Can you work these out from the model? Positions are in its coordinate system, mm. A direction names the side the tool comes from. Round coordinates to 2 decimals unless told otherwise and drop trailing zeros. Order: outer loops, then holes, each group sorted by start corner. A loop starts at its lowest first (then second) coordinate and runs counter-clockwise, first axis right, second up.
Q1. If we section it at B-B (x = -55.5): Please give me the cut outline in (y, z), plus the area to 3 significant figures.
Q2. If we section it at D-D (y = -8.5): Please give me the cut outline in (x, z), plus the area to 3 significant figures.
Q3. If we section it at A-A (z = -10): Please give me the cut outline in (x, y), plus the area to 3 significant figures.
Q4. We'd pull the mould along Y, two halves only. Please class faces 1 (the face through (-21, 82.55, -27)), 2 (the face through (-22, 0, -17)), 3 (the face through (-6, -9, 0)), 4 (the face through (-22, -19.05, -27)): pulls with the +Y half, pulls with the -Y half, needs draft (parallel to the pull), parting line crosses it, or undercut.
Q5. Will these pins go through, and if not, where does the flat tip stop? P1, Ø13.5, axis at x = -21, y = 28.5, coming from the +Z side; P2, Ø6, axis at y = -1, z = -17, coming from the -X side; P3, Ø15, axis at y = 38, z = -31.5, coming from the -X side.
Q6. If I drill on line 1 (Y direction, x = -57.5, z = -32); line 2 (Z direction, x = -14, y = 40.5); line 3 (X direction, y = 16, z = -36.5), over which ranges is the centre line in solid material (lowest first)?
Q7. For faces 5 (the face through (-61.21, -9, -38)), 6 (the face through (-37.912, -9.392, -15.656)), which set-ups out of +Z, -Z, +X, -X, +Y, -Y let a thin tool reach every point of the face, with its end or its side?
Q8. If we section it at C-C (z = -40): Please give me the cut outline in (x, y).
from build123d import *

# Parameters (mm, degrees)
F1_DEPTH = 19.05
F2_W     = 63.5
F2_H     = 19.050002
F3_DEPTH = 44.45
F5_DEPTH = 19.05


with BuildPart() as f1:
    # F0 (on Front) → F1 (new body)
    with BuildSketch(Plane.XZ):
        Polygon((-61.209836, -31.755634), (-61.209836, -44.45), (3.793104, -44.45), (3.793104, 0), (-15.256896, 0), align=None)
    extrude(amount=F1_DEPTH)

    # F2 (on Right) → F3 (join)
    with BuildSketch(Plane.YZ):
        with Locations((31.75, -34.74861)):
            Rectangle(F2_W, F2_H)
    extrude(amount=-F3_DEPTH)

    # F4 (on face) → F5 (join)
    with BuildSketch(Plane(origin=(0, 63.5, 0), x_dir=(-1, 0, 0), z_dir=(0, 1, 0))):
        Polygon((-3.725521, 0), (-3.725521, -44.273611), (61.737206, -44.351444), (61.737206, -32.287851), (15.789114, 0), align=None)
    extrude(amount=F5_DEPTH)


solid = f1.part
Solution:
1. outline: (-19.05, -44.45) - (0, -44.45) - (0, -27.81) - (-19.05, -27.81) - close; (63.5, -44.34) - (82.55, -44.34) - (82.55, -27.9) - (63.5, -27.9) - close
1. area: 630 mm2
2. outline: (-61.21, -44.45) - (3.79, -44.45) - (3.79, 0) - (-15.26, 0) - (-61.21, -31.76) - close
2. area: 2,160 mm2
3. outline: (-30.02, 63.5) - (3.73, 63.5) - (3.73, 82.55) - (-30.02, 82.55) - close; (-29.73, -19.05) - (3.79, -19.05) - (3.79, 0) - (-29.73, 0) - close
3. area: 1,280 mm2
4. face 1: pulls with the +Y half
4. face 2: undercut
4. face 3: needs draft
4. face 4: pulls with the -Y half
5. P1: stops at z = -25.22
5. P2: stops at x = -44.2
5. P3: stops at x = -44.45
6. line 1: y = -19.05 to 0, 63.5 to 82.55
6. line 2: z = -44.27 to -25.22
6. line 3: x = -44.45 to 0
7. face 5: +Z, -Z, -X, -Y
7. face 6: +Z, -X, -Y
8. outline: (-61.74, 63.5) - (-44.45, 63.5) - (-44.45, 0) - (-61.21, 0) - (-61.21, -19.05) - (3.79, -19.05) - (3.79, 0) - (0, 0) - (0, 63.5) - (3.73, 63.5) - (3.73, 82.55) - (-61.74, 82.55) - close
